The model under review builds one solid part; all positions refer to its coordinate system, in mm. A direction names the side the tool comes from. Coordinates: 2 decimals unless noted, no trailing zeros. Loops run counter-clockwise (first coordinate to the right, second up) from the corner with the lowest first, then second, coordinate; pieces in that order, holes last. Notation, with made-up numbers: (60, 25.5) - (64, 25.5) arc R20 cw to (64, 39.5) - close; hole circle Ø1 at (30, 23). An arc over 180 degrees is marked (long way). Answer in a Markdown table with one row per item. Add a question column.
(1) For P1, Ø3.5, axis at y = 17.2, z = 11, coming from the -X side; P2, Ø12, axis at x = 25, z = 5, coming from the +Y side, all flat-tipped, find the tip position at first contact; note any pin that passes through.
(2) Machinability: for faces 1 (the flat face through (17, 11, 0)), 2 (the cylindrical face through (17.224, 5.598, -0.224)), which of the approach directions +Z, -Z, +X, -X, +Y, -Y give a long, thin tool a straight path to every point of the face, cutting with its end or side? Answer none if there is none.
(3) We need section A-A on z = -11. Write out the cut boundary in (x, y), plus the area to 3 significant figures.
(4) For line 1 along Y through (x, z) = (36, 0); line 2 along Y through (x, z) = (35.5, -11); line 3 along Y through (x, z) = (25, 2.5), list the stretches that pass through material, from the lowest coordinate up.
(5) We need section D-D on y = 5.5. Write out the cut boundary in (x, z).
(6) We need section C-C on x = 15. Write out the cut boundary in (y, z), plus the area to 3 significant figures.
(7) We need section B-B on y = 23. Write out the cut boundary in (x, z), plus the area to 4 significant figures.
(8) Mouldability with a two-part tool opening along Y and no side actions: class faces 3 (the cylindrical face through (36.226, 12.994, -2.222)), 4 (the flat face through (36, 61, 0)), 5 (the flat face through (0, 5, 12)) as +Y half, -Y half, draft (parallel to the pull), parting line (faces both ways), or undercut.
from build123d import *

# Parameters (mm, degrees)
BOSS_EXTRUDE1_DEPTH = 11
SKETCH2_W           = 3.5
SKETCH2_H           = 32
BOSS_EXTRUDE2_DEPTH = 50
SKETCH3_R           = 10.25
SKETCH3_R_2         = 1.783609491
SKETCH3_R_3         = 1.426196869
CUT_EXTRUDE1_DEPTH  = 50
SKETCH4_R           = 2.22645949
CUT_EXTRUDE2_DEPTH  = 36


with BuildPart() as part:
    # Sketch1 → Boss-Extrude1 (new body)
    with BuildSketch(Plane(origin=(0, 0, 0), x_dir=(1, 0, 0), z_dir=(0, 1, 0))):
        with BuildLine():
            Line((38, 16), (0, 16))
            Line((0, 16), (0, 7.5))
            ThreePointArc((0, 7.5), (5.303300859, 5.303300859), (7.5, 0))
            ThreePointArc((7.5, 0), (5.303300859, -5.303300859), (0, -7.5))
            Line((0, -7.5), (0, -16))
            Line((0, -16), (38, -16))
            Line((38, -16), (38, 16))
        make_face()
    extrude(amount=BOSS_EXTRUDE1_DEPTH)

    # Sketch2 → Boss-Extrude2 (add)
    with BuildSketch(Plane(origin=(0, 11, 0), x_dir=(1, 0, 0), z_dir=(0, 1, 0))):
        with Locations((36.25, 0)):
            Rectangle(SKETCH2_W, SKETCH2_H)
    extrude(amount=BOSS_EXTRUDE2_DEPTH)

    # Sketch3 → Cut-Extrude1 (cut)
    with BuildSketch(Plane.ZY.offset(-34.5)):
        with Locations((0, 23)):
            Circle(SKETCH3_R)
        with Locations((-11, 17.202811543)):
            Circle(SKETCH3_R_2)
        with Locations((11, 17.202811543)):
            Circle(SKETCH3_R_3)
    extrude(amount=-CUT_EXTRUDE1_DEPTH, mode=Mode.SUBTRACT)

    # Sketch4 → Cut-Extrude2 (cut)
    with BuildSketch(Plane(origin=(0, 0, -16), x_dir=(-1, 0, 0), z_dir=(0, 0, -1))):
        with Locations((-15, 5.5)):
            Circle(SKETCH4_R)
    extrude(amount=-CUT_EXTRUDE2_DEPTH, mode=Mode.SUBTRACT)


solid = part.part
Outcome:
| question | item | result |
|---|---|---|
| 1 | P1 | x = 34.5 |
| 1 | P2 | y = 11 |
| 2 | face 1 | +Z, -Z, -X, +Y |
| 2 | face 2 | +Z, -Z |
| 3 | outline | (0, 0) - (38, 0) - (38, 15.42) - (34.5, 15.42) - (34.5, 11) - (0, 11) - close; (34.5, 18.99) - (38, 18.99) - (38, 61) - (34.5, 61) - close; hole circle Ø4.45 at (15, 5.5) |
| 3 | area | 565 mm² |
| 4 | line 1 | 0 to 12.75, 33.25 to 61 |
| 4 | line 2 | 0 to 15.42, 18.99 to 61 |
| 4 | line 3 | 0 to 11 |
| 5 | outline | (0, -16) - (12.77, -16) - (12.77, 16) - (0, 16) - (0, 7.5) arc R7.5 cw to (0, -7.5) - close; (17.23, -16) - (38, -16) - (38, 16) - (17.23, 16) - close |
| 6 | outline | (0, -16) - (3.27, -16) - (3.27, 16) - (0, 16) - close; (7.73, -16) - (11, -16) - (11, 16) - (7.73, 16) - close |
| 6 | area | 210 mm² |
| 7 | outline | (34.5, -16) - (38, -16) - (38, -10.25) - (34.5, -10.25) - close; (34.5, 10.25) - (38, 10.25) - (38, 16) - (34.5, 16) - close |
| 7 | area | 40.25 mm² |
| 8 | face 3 | undercut |
| 8 | face 4 | +Y half |
| 8 | face 5 | draft |
